CAD build for the part. Positions are in the model's coordinates, mm. Face numbers are marked on the shaded views. A direction names the side the tool comes from. Give positions to 0.01 mm unless a question says otherwise; leave off trailing zeros. Loops run counter-clockwise (first coordinate to the right, second up) from the corner with the lowest first, then second, coordinate; pieces in that order, holes last. Notation, with made-up numbers: M 49.25,-30.75 L 98.25,-30.75 A23 ccw 98.25,-13.75 Z; hole C 84.25,73 d11. An arc over 180 degrees is marked long. One line per question, with ' | ' between items.
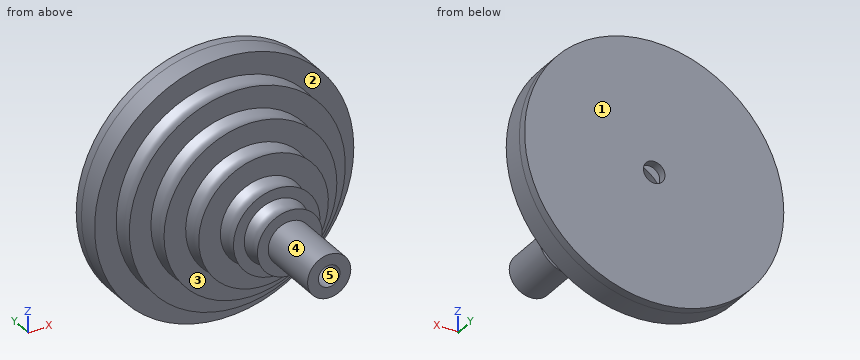
```python
from build123d import *

# Parameters (mm, degrees)
F0_R      = 30
F0_R_2    = 20
F1_DEPTH  = 5
F2_R      = 25
F2_R_2    = 20
F2_R_3    = 15
F3_DEPTH  = 5
F4_R      = 20
F4_R_2    = 15
F4_R_3    = 10
F5_DEPTH  = 5
F6_R      = 15
F6_R_2    = 10
F6_R_3    = 5
F7_DEPTH  = 5
F8_R      = 10
F8_R_2    = 5
F9_DEPTH  = 5
F13_R     = 7.5
F13_R_2   = 5
F13_R_3   = 2.5
F14_DEPTH = 5
F15_R     = 5
F15_R_2   = 2.5
F16_DEPTH = 15
F19_R     = 30
F19_R_2   = 2.5
F20_DEPTH = 2


with BuildPart() as f1:
    # F0 (on Front) → F1 (new body)
    with BuildSketch(Plane.XZ):
        Circle(F0_R)
        Circle(F0_R_2, mode=Mode.SUBTRACT)
    extrude(amount=F1_DEPTH)

    # F2 (on face) → F3 (join)
    with BuildSketch(Plane.XZ.offset(5)):
        Circle(F2_R)
        Circle(F2_R_2, mode=Mode.SUBTRACT)
        Circle(F2_R_2)
        Circle(F2_R_3, mode=Mode.SUBTRACT)
    extrude(amount=F3_DEPTH)

    # F4 (on face) → F5 (join)
    with BuildSketch(Plane.XZ.offset(10)):
        Circle(F4_R)
        Circle(F4_R_2, mode=Mode.SUBTRACT)
        Circle(F4_R_2)
        Circle(F4_R_3, mode=Mode.SUBTRACT)
    extrude(amount=F5_DEPTH)

    # F6 (on face) → F7 (join)
    with BuildSketch(Plane.XZ.offset(15)):
        Circle(F6_R)
        Circle(F6_R_2, mode=Mode.SUBTRACT)
        Circle(F6_R_2)
        Circle(F6_R_3, mode=Mode.SUBTRACT)
    extrude(amount=F7_DEPTH)

    # F8 (on face) → F9 (join)
    with BuildSketch(Plane.XZ.offset(20)):
        Circle(F8_R)
        Circle(F8_R_2, mode=Mode.SUBTRACT)
    extrude(amount=F9_DEPTH)

    # F10 (on Right) → F12 (revolve, cut)
    with BuildSketch(Plane.YZ):
        with BuildLine():
            add(Edge.make_bspline(
                [(-5, 25), (-5.8326505031, 24.531605213), (-7.4963397946, 23.693799982), (-9.1746699077, 24.5308889348), (-10, 25)],
                knots=[0, 0, 0, 0, 0.5, 1, 1, 1, 1], degree=3))
            Line((-5, 25), (-10, 25))
        make_face()
        with BuildLine():
            add(Edge.make_bspline(
                [(-10, 20), (-10.8326505031, 19.531605213), (-12.4963397946, 18.693799982), (-14.1746699077, 19.5308889348), (-15, 20)],
                knots=[0, 0, 0, 0, 0.5, 1, 1, 1, 1], degree=3))
            Line((-10, 20), (-15, 20))
        make_face()
        with BuildLine():
            add(Edge.make_bspline(
                [(-15, 15), (-15.8326505031, 14.531605213), (-17.4963397946, 13.693799982), (-19.1746699077, 14.5308889348), (-20, 15)],
                knots=[0, 0, 0, 0, 0.5, 1, 1, 1, 1], degree=3))
            Line((-15, 15), (-20, 15))
        make_face()
        with BuildLine():
            add(Edge.make_bspline(
                [(-20, 10), (-20.8326505031, 9.531605213), (-22.4963397946, 8.693799982), (-24.1746699077, 9.5308889348), (-25, 10)],
                knots=[0, 0, 0, 0, 0.5, 1, 1, 1, 1], degree=3))
            Line((-20, 10), (-25, 10))
        make_face()
    revolve(axis=Axis((0, 20.6356514245, 0), (0, 1, 0)), mode=Mode.SUBTRACT)

    # F13 (on face) → F14 (join)
    with BuildSketch(Plane.XZ.offset(25)):
        Circle(F13_R)
        Circle(F13_R_2, mode=Mode.SUBTRACT)
        Circle(F13_R_2)
        Circle(F13_R_3, mode=Mode.SUBTRACT)
    extrude(amount=F14_DEPTH)

    # F15 (on face) → F16 (join)
    with BuildSketch(Plane.XZ.offset(30)):
        Circle(F15_R)
        Circle(F15_R_2, mode=Mode.SUBTRACT)
    extrude(amount=F16_DEPTH)

    # F17 (on Right) → F18 (revolve, cut)
    with BuildSketch(Plane.YZ):
        with BuildLine():
            add(Edge.make_bspline(
                [(-25, 7.5), (-25.8326505031, 7.031605213), (-27.4963397946, 6.193799982), (-29.1746699077, 7.0308889348), (-30, 7.5)],
                knots=[0, 0, 0, 0, 0.5, 1, 1, 1, 1], degree=3))
            Line((-25, 7.5), (-30, 7.5))
        make_face()
    revolve(axis=Axis((0, -30.2864443511, 0), (0, -1, 0)), mode=Mode.SUBTRACT)

    # F19 (on face) → F20 (join)
    with BuildSketch(Plane(origin=(0, 0, 0), x_dir=(-1, 0, 0), z_dir=(0, 1, 0))):
        Circle(F19_R)
        Circle(F19_R_2, mode=Mode.SUBTRACT)
    extrude(amount=F20_DEPTH)


solid = f1.part
```
Item 1: Drill centre lines: line 1 along Z through (x, y) = (0, 1.25); line 2 along Y through (x, z) = (13.5, 11); line 3 along Y through (x, z) = (-5, -9). Where is each one in solid material? Low to high. Write a range as [from, to].
Conclusion:
line 1: [-30, -2.5], [2.5, 30] | line 2: [-15, -5], [0, 2] | line 3: [-20, -10], [0, 2]
Item 2: 3-axis set-ups, long thin cutter, end or side, ignore diameter. For the marked faces 1 and 2: which of +Z, -Z, +X, -X, +Y, -Y reach the whole face in a straight line?
Conclusion:
face 1: +Z, -Z, +X, -X, +Y | face 2: -Y
Item 3: Drop flat-ended pins along their axis: P1, Ø6, axis at x = -5.5, y = -39, coming from the -Z side; P2, Ø6, axis at x = 21.5, z = -10, coming from the -Y side; P3, Ø1.5, axis at x = 9, z = -17.5, coming from the -Y side; P4, Ø3, axis at x = 0, z = 0, coming from the -Y side. Give the stop position or say it passes through.
Conclusion:
P1: z = -4.33 | P2: y = -10 | P3: y = -15 | P4: through
Item 4: Saw through at A-A on y = -38. Give the cut face in (x, z).
Conclusion:
outline: C 0,0 d10; hole C 0,0 d5
Item 5: Mould opens along X. For the marked faces 3, 4 and 5 say: pulls with the +X half, pulls with the -X half, needs draft (parallel to the pull), parting line crosses it, or undercut.
Conclusion:
face 3: needs draft | face 4: parting line crosses it | face 5: undercut
